Source: three-view drawing plus pictorial views. Frame: mm from the lowest corner of the part. A direction names the side the tool comes from. Coordinates: 2 decimals unless noted, no trailing zeros. Order: outer loops, then holes, each group sorted by start corner. A loop starts at its lowest first (then second) coordinate and runs counter-clockwise, first axis right, second up. Notation, with made-up numbers: M -10.75,-36 L 3.25,-36 A8 ccw 3.25,-23 Z; hole C -3,9 d5. An arc over 180 degrees is marked long. Use CSV: the item, a comma, the result in double quotes. Start each with the question number.
Q1. Section query B-B, the plane x = 66. Output: boundary loops of the cut face in (y, z).
Q2. Section query A-A, the plane z = 1.5. Output: boundary loops of the cut face in (x, y), and give its area (3 significant figures).
Q3. Mould query, pull axis Y, two halves, no side actions, for the marked faces 4, 5 and 6. Classes: +Y half, -Y half, draft (parallel to the pull), parting line (faces both ways), or undercut.
Q4. Access query for the marked faces 1, 2 and 3. Directions: +Z, -Z, +X, -X, +Y, -Y. A direction counts if a zero-diameter tool reaches every point of the face in a straight line with its end or side. Return the directions, or none.
Q5. Section query C-C, the plane y = 10. Output: boundary loops of the cut face in (x, z) (3 decimals), and give its area (3 significant figures).
Q6. Ray query, probe 1 along X at (y, z) = (10, 6); probe 2 along Y at (x, z) = (10, 7.5); probe 3 along Z at (x, y) = (39, 2) (3 decimals). Return the intervals inside material, ascending.
Q7. First-contact query: P1, Ø5.5, axis at x = 10, y = 10, coming from the +Z side; P2, Ø10, axis at x = 37, y = 9, coming from the -Z side (3 decimals); P3, Ø1.7, axis at x = 35.5, y = 16, coming from the -Z side. Flat tips, straight axial feed; report the tip coordinate or a pass-through.
Q8. Section query D-D, the plane y = 1.5. Output: boundary loops of the cut face in (x, z) (3 decimals), and give its area (3 significant figures).
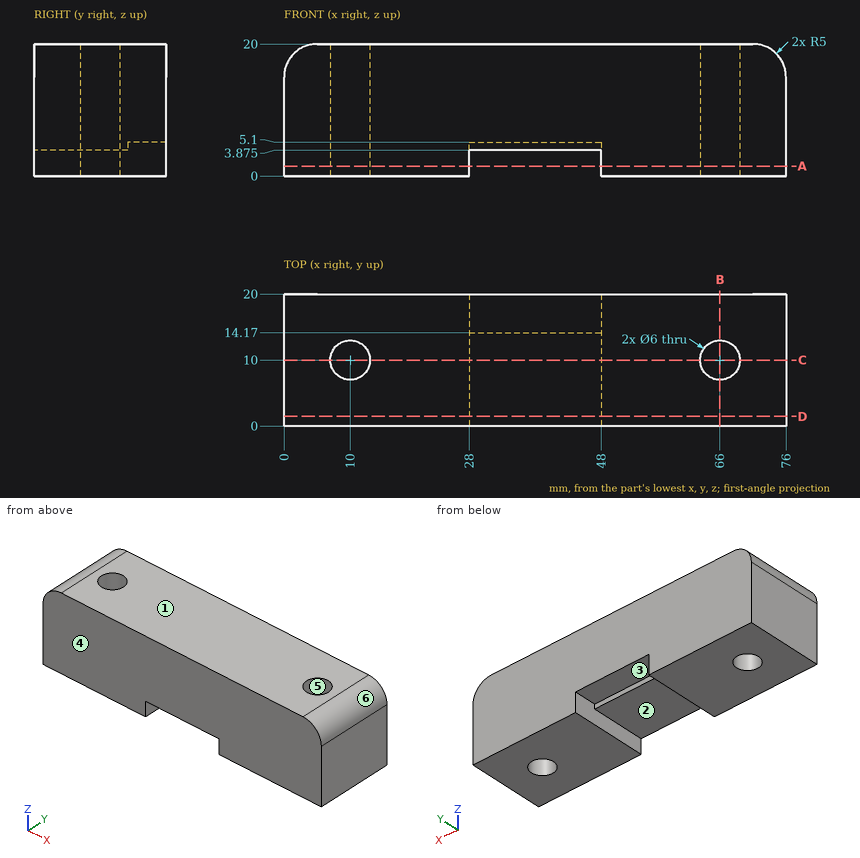
Responses:
1,outline,"M 0,0 L 7,0 L 7,20 L 0,20 Z; M 13,0 L 20,0 L 20,20 L 13,20 Z"
2,outline,"M 0,0 L 28,0 L 28,20 L 0,20 Z; M 48,0 L 76,0 L 76,20 L 48,20 Z; hole C 10,10 d6; hole C 66,10 d6"
2,area,"1,060 mm²"
3,face 4,"-Y half"
3,face 5,"undercut"
3,face 6,"draft"
4,face 1,"+Z, +X, -X, +Y, -Y"
4,face 2,"-Z, +Y, -Y"
4,face 3,"-Z, +Y"
5,outline,"M 0,0 L 7,0 L 7,20 L 5,20 A5 ccw 0,15 Z; M 13,0 L 28,0 L 28,3.875 L 48,3.875 L 48,0 L 63,0 L 63,20 L 13,20 Z; M 69,0 L 76,0 L 76,15 A5 ccw 71,20 L 69,20 Z"
5,area,"1,190 mm²"
6,probe 1,"x = 0 to 7, 13 to 63, 69 to 76"
6,probe 2,"y = 0 to 7, 13 to 20"
6,probe 3,"z = 3.875 to 20"
7,P1,"passes through"
7,P2,"stops at z = 3.875"
7,P3,"stops at z = 5.1"
8,outline,"M 0,0 L 28,0 L 28,3.875 L 48,3.875 L 48,0 L 76,0 L 76,15 A5 ccw 71,20 L 5,20 A5 ccw 0,15 Z"
8,area,"1,430 mm²"
